Autodesk Inventor part; units mm, degrees
ref_plane "YZ Plane" through (0, 0, 0) normal (1, 0, 0) x (0, 1, 0)
ref_plane "XZ Plane" through (0, 0, 0) normal (0, 1, 0) x (-1, 0, 0)
ref_plane "XY Plane" through (0, 0, 0) normal (0, 0, 1) x (1, 0, 0)
sketch "Sketch1" plane through (0, 0, 0) normal (0, 0, 1) x (1, 0, 0)
  circle A0 centre (-13, 0) radius 1
  circle A1 centre (13, 0) radius 1
  circle A2 centre (-13, 0) radius 4
  circle A3 centre (13, 0) radius 4
  point P0 (0, 0)
  dimension "d0" = 2
  dimension "d1" = 2
  dimension "d3" = 26
  dimension "d4" = 13
  dimension "d5" = 8
  dimension "d6" = 8
extrude "Extrusion1" add sketch "Sketch1" against normal mid plane 18
sketch "Sketch2" plane through (0, 0, 0) normal (0, 0, 1) x (1, 0, 0)
  circle A0 centre (-13, 0) radius 4
  circle A1 centre (-13, 0) radius 1
  point P0 (0, 0)
extrude "Extrusion2" cut sketch "Sketch2" against normal mid plane 9
sketch "Sketch3" plane through (-13, 0, -4.5) normal (0, 0, 1) x (1, 0, 0)
  circle A0 centre (26, 0) radius 4
  circle A1 centre (26, 0) radius 4
  circle A2 centre (26, 0) radius 1
  point P0 (13, 0)
extrude "Extrusion3" cut sketch "Sketch3" against normal blind 4.5
mirror "Mirror1" about plane through (0, 0, 0) normal (0, 0, 1) of "Extrusion3"
sketch "Sketch6" plane through (0, 0, 0) normal (0, 1, 0) x (-1, 0, 0)
  line L0 (-9, -4.5) -> (-12, -4.5) construction
  line L1 (-12, -4.5) -> (-12, 4.5) construction
  line L2 (-12, 4.5) -> (-9, 4.5) construction
  line L3 (-9, 4.5) -> (-9, -4.5) construction
  line L4 (-14, -4.5) -> (-17, -4.5) construction
  line L5 (-17, -4.5) -> (-17, 4.5) construction
  line L6 (-17, 4.5) -> (-14, 4.5) construction
  line L7 (-14, 4.5) -> (-14, -4.5) construction
  line L8 (9, 9) -> (12, 9) construction
  line L9 (12, 9) -> (12, 4.5) construction
  line L10 (12, 4.5) -> (9, 4.5) construction
  line L11 (9, 4.5) -> (9, 9) construction
  line L12 (14, 9) -> (17, 9) construction
  line L13 (17, 9) -> (17, 4.5) construction
  line L14 (17, 4.5) -> (14, 4.5) construction
  line L15 (14, 4.5) -> (14, 9) construction
  line L16 (17, -9) -> (14, -9) construction
  line L17 (14, -9) -> (14, -4.5) construction
  line L18 (14, -4.5) -> (17, -4.5) construction
  line L19 (17, -4.5) -> (17, -9) construction
  line L20 (12, -9) -> (9, -9) construction
  line L21 (9, -9) -> (9, -4.5) construction
  line L22 (9, -4.5) -> (12, -4.5) construction
  line L23 (12, -4.5) -> (12, -9) construction
  line L24 (9, -9) -> (17, -9) construction
  line L25 (9, -9) -> (6, -9)
  line L26 (6, -9) -> (6, -2)
  line L27 (6, -2) -> (-9, -2)
  line L28 (-9, 4.5) -> (-9, -4.5) construction
  line L29 (-9, 2) -> (6, 2)
  line L30 (6, 2) -> (6, 9)
  line L31 (6, 9) -> (9, 9)
  line L32 (9, -4.5) -> (17, -4.5) construction
  line L33 (9, -4.5) -> (9, 4.5)
  line L34 (-9, -2) -> (-12, -2)
  line L35 (-12, -4.5) -> (-12, 4.5)
  line L36 (-9, 2) -> (-12, 2)
  line L37 (9, -9) -> (12, -9)
  line L38 (12, -4.5) -> (9, -4.5)
  line L39 (14, -4.5) -> (12, -4.5)
  line L40 (12, -4.5) -> (12, -9)
  line L41 (12, -9) -> (12, -4.5)
  line L42 (12, 4.5) -> (14, 4.5)
  line L43 (17, 4.5) -> (9, 4.5)
  line L44 (12, 4.5) -> (9, 4.5)
  line L45 (12, 9) -> (14, 9)
  line L46 (12, 4.5) -> (12, 9)
  line L47 (17, 9) -> (9, 9)
  line L48 (12, 9) -> (9, 9)
  point P0 (0, 0)
  dimension "d16" = 3
  dimension "d17" = 4
  dimension "d18" = 2
extrude "Extrusion4" add sketch "Sketch6" against normal mid plane 4
sketch "Sketch7" plane through (-9, -2, -4.5) normal (-1, 0, 0) x (0, 0, 1)
  circle A0 centre (4.5, 2) radius 1
  dimension "d21" = 2
extrude "Extrusion5" cut sketch "Sketch7" against normal blind 20
chamfer "Chamfer1" distance 1 angle 45 1 edges at (-9, 0, -1)
fillet "Fillet1" radius 2 4 edges at (1.7679, 2, 2) (1.7679, 2, -2) (1.7679, -2, -2) (1.7679, -2, 2)
sketch "Sketch9" plane through (0, 0, 9) normal (0, 0, 1) x (1, 0, 0)
  circle A0 centre (-13, 0) radius 1
  circle A1 centre (-13, 0) radius 0.9
  point P0 (0, 0)
  dimension "d29" = 1.8
extrude "TREAD" add sketch "Sketch9" against normal up to surface (4.5 mm away)
sketch "Sketch11" plane through (13, 0, 4.5) normal (0, 0, 1) x (1, 0, 0)
  circle A0 centre (0, 0) radius 4
  circle A1 centre (0, 0) radius 1
  point P0 (-13, 0)
extrude "thin" cut sketch "Sketch11" against normal blind 0.1
mirror "Mirror2" about plane through (0, 0, 0) normal (0, 0, 1) of "thin"
sketch "Sketch12" plane through (13, 0, 4.4) normal (0, 0, 1) x (1, 0, 0)
  circle A0 centre (0, 0) radius 1 construction
  circle A1 centre (0, 0) radius 1.1
  point P0 (-13, 0)
  dimension "d34" = 2.2
extrude "Extrusion8" cut sketch "Sketch12" against normal up to surface (8.8 mm away)
equation "\"d6\" = d5"
properties part number "tOLERNECED_Phalalnge_28mm"
Model file for the job. Use its own axes, mm. A direction names the side the tool comes from. Coordinates: 2 decimals unless noted, no trailing zeros. Loops run counter-clockwise (first coordinate to the right, second up) from the corner with the lowest first, then second, coordinate; pieces in that order, holes last. Notation, with made-up numbers: M -4,-30 L 40,-30 A12 ccw 40,-23 Z; hole C 71.5,-21 d5. An arc over 180 degrees is marked long. Use CSV: the item, a comma, the result in double quotes. Start each with the question number.
1. Probe probe 1 along Y at (x, z) = (1, 0); probe 2 along X at (y, z) = (0.25, 3); probe 3 along Y at (x, z) = (13, 4). List the from-to ranges inside material, lowest first. Write a range as [from, to].
2. Band-saw the part on A-A, the plane z = -3.75. List the corners of the cut face in (x, y), then the cut area to 3 significant figures.
3. Band-saw the part on C-C, the plane x = -13. List the corners of the cut face in (y, z).
4. Band-saw the part on D-D, the plane y = -2.5. List the corners of the cut face in (x, z).
5. Tool access for faces 1 (the cylindrical face through (1.88, 1.43, 1.4)), 2 (the flat face through (12, -1, -4.4)), 3 (the cylindrical face through (1.88, -1.43, -1.4)), 4 (the flat face through (-8, -2, 0)), 5 (the cylindrical face through (1.88, 1.4, -1.43)): list every direction of +Z, -Z, +X, -X, +Y, -Y with a clear straight run to the whole face (end or side of a thin tool).
6. Two-plate mould, pull along Y, no slides. Class faces 6 (the cylindrical face through (1.66, -1.43, 1.4)), 7 (the flat face through (-12, -1, -4.5)), 8 (the cylindrical face through (12.13, -0.67, 0.06)): pulls with the +Y half, pulls with the -Y half, needs draft (parallel to the pull), parting line crosses it, or undercut.
7. Flat gauge pins, fed straight in: pin 1 (1.6 mm diameter, centred on x = -13, y = 0, fed in from -Z); pin 2 (4 mm diameter, centred on x = 14.5, y = -2, fed in from +Z); pin 3 (4 mm diameter, centred on x = -5.5, z = 5, fed in from +Y); pin 4 (1 mm diameter, centred on y = -0.5, z = -0.5, fed in from -X). Where does each tip first touch, or does it go through?
8. Band-saw the part on B-B, the plane x = 13. List the corners of the cut face in (y, z).
Entries:
1,probe 1,"y = [-2, -1], [1, 2]"
1,probe 2,"x = [-9, -6], [9.01, 11.93], [14.07, 16.99]"
1,probe 3,"y = [-4, -1.1], [1.1, 4]"
2,outline,"M -9,-2 L -6,-2 L -6,2 L -9,2 Z; C 13,0 d8; hole C 13,0 d2.2"
2,area,"58.5 mm2"
3,outline,"M -4,-9 L -1,-9 L -1,-4.5 L -4,-4.5 Z; M -4,4.5 L -0.9,4.5 L -0.9,9 L -4,9 Z; M 0.9,4.5 L 4,4.5 L 4,9 L 0.9,9 Z; M 1,-9 L 4,-9 L 4,-4.5 L 1,-4.5 Z"
4,outline,"M -16.12,-9 L -9.88,-9 L -9.88,-4.5 L -16.12,-4.5 Z; M -16.12,4.5 L -9.88,4.5 L -9.88,9 L -16.12,9 Z; M 9.88,-4.4 L 16.12,-4.4 L 16.12,4.4 L 9.88,4.4 Z"
5,face 1,"+Z, +Y"
5,face 2,"-Z, +X, +Y, -Y"
5,face 3,"-Z, -Y"
5,face 4,"+Z, -Z, -Y"
5,face 5,"-Z, +Y"
6,face 6,"pulls with the -Y half"
6,face 7,"needs draft"
6,face 8,"undercut"
7,pin 1,"passes through"
7,pin 2,"stops at z = 4.4"
7,pin 3,"stops at y = 2"
7,pin 4,"stops at x = -8.21"
8,outline,"M -4,-4.4 L -1.1,-4.4 L -1.1,4.4 L -4,4.4 Z; M 1.1,-4.4 L 4,-4.4 L 4,4.4 L 1.1,4.4 Z"
